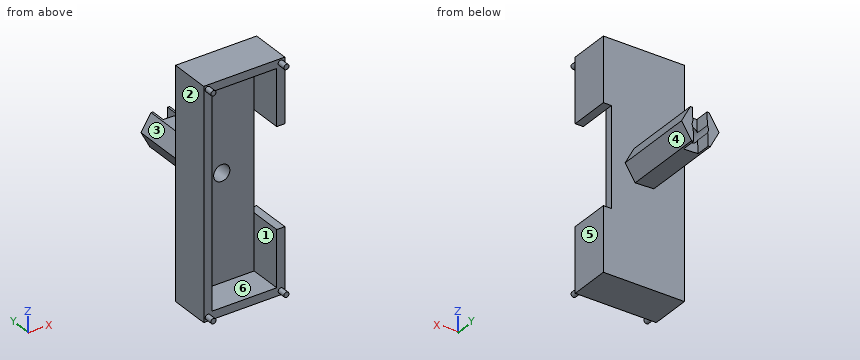
Autodesk Inventor part; units mm, degrees
ref_plane "YZ Plane" through (0, 0, 0) normal (1, 0, 0) x (0, 1, 0)
ref_plane "XZ Plane" through (0, 0, 0) normal (0, 1, 0) x (-1, 0, 0)
ref_plane "XY Plane" through (0, 0, 0) normal (0, 0, 1) x (1, 0, 0)
sketch "Sketch1" plane through (0, 0, 0) normal (0, 1, 0) x (-1, 0, 0)
  point P0 (0, 0)
sketch "Sketch2" plane through (0, 0, 0) normal (0, 1, 0) x (-1, 0, 0)
  line L0 (11.0402, 14.5) -> (-38.9598, 14.5)
  line L1 (-38.9598, -125.5) -> (11.0402, -125.5)
  line L2 (11.0402, -125.5) -> (11.0402, 14.5)
  line L3 (-38.9598, -25) -> (-33.9598, -25)
  line L4 (-38.9598, -86) -> (-33.9598, -86)
  line L5 (-38.9598, 14.5) -> (-38.9598, -25)
  line L6 (-38.9598, -86) -> (-38.9598, -125.5)
  line L7 (-33.9598, -25) -> (-33.9598, 9.5)
  line L8 (-33.9598, 9.5) -> (6.0402, 9.5)
  line L9 (6.0402, 9.5) -> (6.0402, -120.5)
  line L10 (6.0402, -120.5) -> (-33.9598, -120.5)
  line L11 (-33.9598, -120.5) -> (-33.9598, -86)
  point P0 (0, 0)
  dimension "d0" = 50
  dimension "d1" = 140
  dimension "d2" = 5
  dimension "d3" = 39.5
  dimension "d4" = 39.5
  dimension "d5" = 34.5
  dimension "d6" = 40
  dimension "d7" = 130
extrude "Extrusion1" add sketch "Sketch2" along normal blind 20
sketch "Sketch3" plane through (0, 20, 0) normal (0, 1, 0) x (1, 0, 0)
  line L0 (-11.0402, 125.5) -> (-11.0402, -14.5)
  line L1 (38.9598, 125.5) -> (-11.0402, 125.5)
  line L2 (-11.0402, -14.5) -> (38.9598, -14.5)
  line L3 (38.9598, 125.5) -> (-11.0402, 125.5)
  line L4 (-11.0402, 125.5) -> (-11.0402, -14.5)
  line L5 (33.9598, 86) -> (38.9598, 86)
  line L6 (38.9598, 25) -> (33.9598, 25)
  line L7 (33.9598, 25) -> (33.9598, -9.5)
  line L8 (33.9598, 25) -> (33.9598, 86)
  line L9 (38.9598, -14.5) -> (38.9598, 25)
  line L10 (38.9598, 86) -> (38.9598, 125.5)
  point P0 (0, 0)
extrude "Extrusion2" add sketch "Sketch3" along normal blind 5
sketch "Sketch4" plane through (0, 25, 0) normal (0, 1, 0) x (1, 0, 0)
  circle A0 centre (13.9598, 55.5) radius 5
  line L0 (-11.0402, -14.5) -> (38.9598, -14.5)
  line L1 (38.9598, 86) -> (38.9598, 125.5)
  point P0 (0, 0)
  dimension "d12" = 10
  dimension "d13" = 70
  dimension "d14" = 25
extrude "Extrusion3" cut sketch "Sketch4" against normal blind 5
sketch "Sketch5" plane through (0, 0, 0) normal (0, -1, 0) x (1, 0, 0)
  circle A0 centre (36.4598, 12) radius 1.6
  line L0 (38.9598, 14.5) -> (38.9598, -25)
  line L1 (-11.0402, 14.5) -> (38.9598, 14.5)
  circle A1 centre (36.4598, -123) radius 1.6
  line L2 (38.9598, -125.5) -> (-11.0402, -125.5)
  line L3 (38.9598, -86) -> (38.9598, -125.5)
  circle A2 centre (-8.5402, -123) radius 1.6
  line L4 (-11.0402, -125.5) -> (-11.0402, 14.5)
  circle A3 centre (-8.5402, 12) radius 1.6
  point P0 (0, 0)
  dimension "d17" = 3.2
  dimension "d18" = 2.5
  dimension "d19" = 2.5
  dimension "d20" = 3.2
  dimension "d21" = 2.5
  dimension "d22" = 2.5
  dimension "d23" = 3.2
  dimension "d24" = 2.5
  dimension "d25" = 2.5
  dimension "d26" = 3.2
  dimension "d27" = 2.5
  dimension "d28" = 2.5
extrude "Extrusion4" add sketch "Sketch5" along normal blind 5
sketch "Sketch6" plane through (0, 25, 0) normal (0, 1, 0) x (1, 0, 0)
  circle A0 centre (13.9598, 55.5) radius 5
  line L0 (8.5818, 45.2818) -> (2.4216, 55.0484)
  line L1 (2.4216, 55.0484) -> (7.7996, 65.2665)
  line L2 (7.7996, 65.2665) -> (19.3378, 65.7182)
  line L3 (19.3378, 65.7182) -> (25.498, 55.9516)
  line L4 (25.498, 55.9516) -> (20.12, 45.7335)
  line L5 (20.12, 45.7335) -> (8.5818, 45.2818)
  point P0 (0, 0)
  dimension "d31" = 10
extrude "Extrusion5" add sketch "Sketch6" along normal blind 50
sketch "Sketch7" plane through (20.12, 25, -45.7335) normal (0.0391109, 0, 0.9992349) x (0.9992349, 0, -0.0391109)
  point P0 (-21.8933, -25)
sketch "Sketch8" plane through (20.12, 25, -45.7335) normal (0.0391109, 0, 0.9992349) x (0.9992349, 0, -0.0391109)
  line L0 (-10.7735, 50) -> (-0.7735, 50)
  line L1 (-10.273, 50) -> (-1.273, 50)
  line L2 (-1.273, 50) -> (-1.273, 41)
  line L3 (-1.273, 41) -> (-10.273, 41)
  line L4 (-10.273, 41) -> (-10.273, 50)
  line L5 (0, 0) -> (0, 50)
  line L6 (-11.547, 0) -> (-11.547, 50)
  point P0 (-21.8933, -25)
  point P1 (-1.273, 50)
  dimension "d34" = 9
  dimension "d35" = 9
  dimension "d36" = 1.273
  dimension "d37" = 1.274
extrude "Extrusion6" cut sketch "Sketch8" against normal through all
properties part number "Caja_Antena"
Geometry: final body of the model. Coordinates: model frame, mm. Face numbers are marked on the shaded views. A direction names the side the tool comes from. Round coordinates to 2 decimals unless told otherwise and drop trailing zeros. Write each loop counter-clockwise with the first axis right and the second up, starting at its lowest first coordinate (ties: lowest second). Pieces come first, ordered by that corner, then holes.
Item 1: Set-up query: the marked faces 1 and 2. Return all of +Z, -Z, +X, -X, +Y, -Y with unobstructed straight access to the full face (end or side cutting, diameter ignored); none if empty.
Item 2: Material intervals for L1, parallel to Z at x = 35, y = 6; L2, parallel to X at y = 39, z = -55; L3, parallel to Z at x = -4, y = 13, sorted ascending.
Item 3: Pin query (flat end, axial travel): P1, Ø1.5, axis at x = 10, y = 65, coming from the -Z side; P2, Ø3, axis at x = 20, z = -16, coming from the +Y side; P3, Ø10, axis at y = 8, z = -37.5, coming from the +X side; P4, Ø6, axis at x = 13.96, z = -55.5, coming from the -Y side. Return the tip coordinate at first contact, or that it passes through.
Item 4: Section query A-A (y = 68.5). Return loops of the section in (x, z), plus the area to 3 significant figures.
Item 5: Section query B-B (z = 12). Return loops of the section in (x, y), plus the area to 3 significant figures.
Item 6: Section query D-D (y = 29). Return loops of the section in (x, z).
Item 7: Section query C-C (x = 11.5). Return loops of the section in (y, z).
Item 8: Mould query, pull axis Z, two halves, no side actions, for the marked faces 3, 4, 5 and 6. Classes: +Z half, -Z half, draft (parallel to the pull), parting line (faces both ways), or undercut.
Completed:
1. face 1: -Y
1. face 2: +Z, -Z, -X, +Y, -Y
2. L1: z = -125.5 to -86, -25 to 14.5
2. L2: x = 2.45 to 8.98, 18.93 to 25
2. L3: z = -125.5 to -120.5, 9.5 to 14.5
3. P1: stops at z = -65.38
3. P2: stops at y = 25
3. P3: stops at x = -6.04
3. P4: passes through
4. outline: (2.42, -55.05) - (7.8, -65.27) - (9.07, -65.32) - (9.38, -57.5) arc R5 cw to (9.55, -53.15) - (9.85, -45.33) - (8.58, -45.28) - close; (18.07, -65.67) - (19.34, -65.72) - (25.5, -55.95) - (20.12, -45.73) - (18.85, -45.68) - (18.54, -53.5) arc R5 cw to (18.37, -57.85) - close
4. area: 163 mm2
5. outline: (-11.04, 0) - (-10.14, 0) - (-10.14, -5) - (-6.94, -5) - (-6.94, 0) - (34.86, 0) - (34.86, -5) - (38.06, -5) - (38.06, 0) - (38.96, 0) - (38.96, 25) - (-11.04, 25) - close
5. area: 1,280 mm2
6. outline: (2.42, -55.05) - (7.8, -65.27) - (19.34, -65.72) - (25.5, -55.95) - (20.12, -45.73) - (8.58, -45.28) - close; hole circle Ø10 at (13.96, -55.5)
7. outline: (0, -125.5) - (25, -125.5) - (25, -65.41) - (66, -65.41) - (66, -59.85) - (20, -59.85) - (20, -120.5) - (0, -120.5) - close; (0, 9.5) - (20, 9.5) - (20, -51.15) - (66, -51.15) - (66, -45.4) - (25, -45.4) - (25, 14.5) - (0, 14.5) - close
8. face 3: +Z half
8. face 4: -Z half
8. face 5: draft
8. face 6: undercut
